Geometry check sheet. Reference: the model listing, model coordinates, mm. Face numbers are marked on the shaded views. A direction names the side the tool comes from. Give positions to 0.01 mm unless a question says otherwise; leave off trailing zeros. Loops run counter-clockwise (first coordinate to the right, second up) from the corner with the lowest first, then second, coordinate; pieces in that order, holes last. Notation, with made-up numbers: (6, -26) -> (43, -26) arc R26 cw to (43, 1) -> close; hole circle Ø9 at (-3.5, 88.5). An arc over 180 degrees is marked (long way). One line per question, with ' | ' between items.
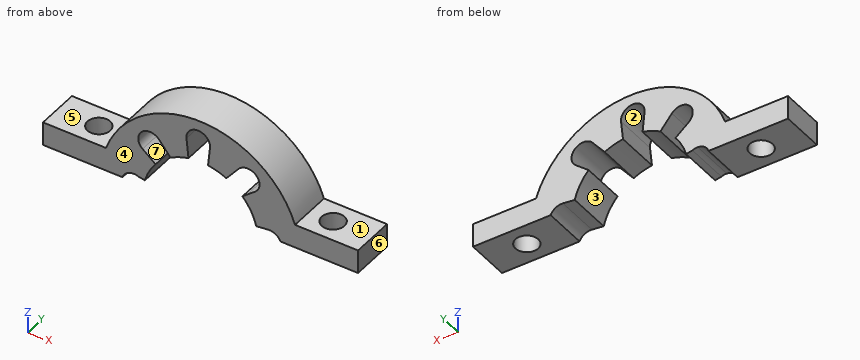
from build123d import *

# Parameters (mm, degrees)
F1_DEPTH = 5.5
F2_R     = 1.45
F3_DEPTH = 25
F4_R     = 1.45
F5_DEPTH = 25


# Not quite as in the source:
# - a feature names something its author has since deleted; it is built from what else it names


with BuildPart() as f1:
    # F0 (on Front) → F1 (new body)
    with BuildSketch(Plane.XZ):
        with BuildLine():
            Line((10.1409122915, -7.7475719752), (20, -7.7475719752))
            Line((20, -7.7475719752), (20, -4.7475719752))
            Line((20, -4.7475719752), (12, -4.7475719752))
            ThreePointArc((12, -4.7475719752), (0, 3.8721859892), (-12, -4.7475719752))
            Line((-12, -4.7475719752), (-20, -4.7475719752))
            Line((-20, -4.7475719752), (-20, -7.7475719752))
            Line((-20, -7.7475719752), (-10, -7.7475719752))
            Line((-10, -7.7475719752), (-9.9101597832, -7.7475719752))
            ThreePointArc((-9.9101597832, -7.7475719752), (-9.399666092, -6.9954026392), (-8.5485111922, -6.6761882044))
            ThreePointArc((-8.5485111922, -6.6761882044), (-8.20089019, -6.698967849), (-7.8678987383, -6.8013200176))
            Line((-7.8678987383, -6.8013200176), (-7.0639233089, -6.9491323338))
            ThreePointArc((-7.0639233089, -6.9491323338), (-6.5280807154, -5.5234621099), (-5.7080769948, -4.2400070969))
            Line((-5.7080769948, -4.2400070969), (-7.3540770708, -2.8946497535))
            ThreePointArc((-7.3540770708, -2.8946497535), (-7.4654597138, -0.6725800185), (-5.2433899789, -0.7839626615))
            Line((-5.2433899789, -0.7839626615), (-3.7957894574, -2.5550538739))
            ThreePointArc((-3.7957894574, -2.5550538739), (-2.6997185699, -2.0081537307), (-1.5276324855, -1.6522248506))
            Line((-1.5276324855, -1.6522248506), (-1.7831469906, 0.8901123752))
            ThreePointArc((-1.7831469906, 0.8901123752), (-0.2906658349, 2.5401123752), (1.2018153207, 0.8901123752))
            Line((1.2018153207, 0.8901123752), (0.9562236033, -1.55349436))
            ThreePointArc((0.9562236033, -1.55349436), (2.1490849475, -1.8141042253), (3.281823707, -2.2698877168))
            Line((3.281823707, -2.2698877168), (4.832326413, -0.3728990956))
            ThreePointArc((4.832326413, -0.3728990956), (7.0560350494, -0.2631578905), (6.9394170389, -2.4865164921))
            Line((6.9394170389, -2.4865164921), (5.9372443956, -3.3004847472))
            Line((5.9372443956, -3.3004847472), (5.3253136848, -3.7974970895))
            ThreePointArc((5.3253136848, -3.7974970895), (6.4103242472, -5.2980690002), (7.0828602188, -7.0233687847))
            Line((7.0828602188, -7.0233687847), (8.5816167977, -6.8438853729))
            ThreePointArc((8.5816167977, -6.8438853729), (9.5121128892, -7.0354424826), (10.1409122915, -7.7475719752))
        make_face()
    extrude(amount=F1_DEPTH)

    # F2 (on face) → F3 (cut)
    with BuildSketch(Plane.XY.offset(-4.7475719752)):
        with Locations((-14.75, -2.75)):
            Circle(F2_R)
    extrude(amount=-F3_DEPTH, mode=Mode.SUBTRACT)

    # F4 (on face) → F5 (cut)
    with BuildSketch(Plane.XY.offset(-4.7475719752)):
        with Locations((15, -2.75)):
            Circle(F4_R)
    extrude(amount=-F5_DEPTH, mode=Mode.SUBTRACT)


solid = f1.part
Item 1: Set-up check for the marked faces 1, 2, 3 and 4: record each of +Z, -Z, +X, -X, +Y, -Y from which the full face is reachable in a straight line by a thin tool's end or side.
Result:
face 1: +Z, +X, +Y, -Y | face 2: +Y, -Y | face 3: -Z, +Y, -Y | face 4: +Z, -Z, +X, -X, -Y
Item 2: Scan lines: probe 1 along Y at (x, z) = (-14.75, -6.25); probe 2 along X at (y, z) = (-0.6, -1); probe 3 along X at (y, z) = (-4, -1.5). Record each from-to range of solid material in increasing order.
Result:
probe 1: -5.5 to -4.2, -1.3 to 0 | probe 2: -9.98 to -7.71, -5.07 to -1.59, 1.01 to 4.32, 7.46 to 9.98 | probe 3: -10.35 to -7.89, -4.66 to -1.54, 0.96 to 3.91, 7.48 to 10.35
Item 3: Sectioned sample at B-B (y = -2.75). Give the number of separate pieces and of enclosed holes in the cut face, plus the area to 3 significant figures.
Result:
separate pieces: 3 | enclosed holes: 0 | area: 150 mm2
Item 4: Depth check by flat-ended pin: pin 1 Ø1.5 at (y, z) = (-2, -1) entering from +X (3 decimals); pin 2 Ø2 at (y, z) = (-3, -3) entering from +X; pin 3 Ø3 at (x, y) = (15, -2.5) entering from +Z. Enter the tip coordinate at first touch or a pass-through.
Result:
pin 1: x = 10.525 | pin 2: x = 11.72 | pin 3: z = -4.75
Item 5: Release check for a two-part mould opening along X. For the marked faces 5, 6 and 7 record: pulls with the +X half, pulls with the -X half, needs draft (parallel to the pull), parting line crosses it, or undercut.
Result:
face 5: needs draft | face 6: pulls with the +X half | face 7: undercut
Item 6: Sectioned sample at D-D (y = -4.7). Record the cut outline in (x, z), plus the area to 3 significant figures.
Result:
outline: (-20, -7.75) -> (-9.91, -7.75) arc R1.5 cw to (-7.87, -6.8) -> (-7.06, -6.95) arc R7.3 cw to (-5.71, -4.24) -> (-7.35, -2.89) arc R1.5 cw (long way) to (-5.24, -0.78) -> (-3.8, -2.56) arc R7.3 cw to (-1.53, -1.65) -> (-1.78, 0.89) arc R1.5 cw (long way) to (1.2, 0.89) -> (0.96, -1.55) arc R7.3 cw to (3.28, -2.27) -> (4.83, -0.37) arc R1.5 cw (long way) to (6.94, -2.49) -> (5.33, -3.8) arc R7.3 cw to (7.08, -7.02) -> (8.58, -6.84) arc R1.5 cw to (10.14, -7.75) -> (20, -7.75) -> (20, -4.75) -> (12, -4.75) arc R12.66 ccw to (-12, -4.75) -> (-20, -4.75) -> close | area: 168 mm2
Item 7: Sectioned sample at C-C (z = -5.25). Record the cut outline in (x, y), plus the area to 3 significant figures.
Result:
outline: (-20, -5.5) -> (-6.38, -5.5) -> (-6.38, 0) -> (-20, 0) -> close; (6.38, -5.5) -> (20, -5.5) -> (20, 0) -> (6.38, 0) -> close; hole circle Ø2.9 at (-14.75, -2.75); hole circle Ø2.9 at (15, -2.75) | area: 137 mm2
Item 8: Sectioned sample at A-A (x = 15). Record the cut outline in (y, z).
Result:
outline: (-5.5, -7.75) -> (-4.2, -7.75) -> (-4.2, -4.75) -> (-5.5, -4.75) -> close; (-1.3, -7.75) -> (0, -7.75) -> (0, -4.75) -> (-1.3, -4.75) -> close
